```python
from build123d import *

# Parameters (mm, degrees)
SKETCH_R      = 1.5
SKETCH_W      = 56
SKETCH_H      = 40
PAD_DEPTH     = 3
SKETCH001_R   = 3
SKETCH001_R_2 = 1.5
PAD001_DEPTH  = 6
SKETCH002_R   = 2.25
POCKET_DEPTH  = 1.5


with BuildPart() as part:
    # Sketch → Pad (new body)
    with BuildSketch(Plane.XY):
        with BuildLine():
            Line((58, -3), (-4, -3))
            ThreePointArc((-7, 0), (-6.12132, -2.12132), (-4, -3))
            Line((-7, 0), (-7, 79))
            ThreePointArc((-1, 79), (-4, 82), (-7, 79))
            Line((-1, 79), (-1, 52))
            Line((-1, 52), (45, 52))
            Line((45, 52), (45, 79))
            ThreePointArc((51, 79), (48, 82), (45, 79))
            Line((51, 79), (51, 52))
            Line((51, 52), (58, 52))
            ThreePointArc((61, 49), (60.12132, 51.12132), (58, 52))
            Line((61, 0), (61, 49))
            ThreePointArc((58, -3), (60.12132, -2.12132), (61, 0))
        make_face()
        Circle(SKETCH_R, mode=Mode.SUBTRACT)
        with Locations((58, 0)):
            Circle(SKETCH_R, mode=Mode.SUBTRACT)
        with Locations((0, 49)):
            Circle(SKETCH_R, mode=Mode.SUBTRACT)
        with Locations((58, 49)):
            Circle(SKETCH_R, mode=Mode.SUBTRACT)
        with Locations((-4, 3)):
            Circle(SKETCH_R, mode=Mode.SUBTRACT)
        with Locations((48, 3)):
            Circle(SKETCH_R, mode=Mode.SUBTRACT)
        with Locations((48, 79)):
            Circle(SKETCH_R, mode=Mode.SUBTRACT)
        with Locations((-4, 79)):
            Circle(SKETCH_R, mode=Mode.SUBTRACT)
        with Locations((27, 26)):
            Rectangle(SKETCH_W, SKETCH_H, mode=Mode.SUBTRACT)
    extrude(amount=PAD_DEPTH)

    # Sketch001 (on Face27 of Pad) → Pad001 (join)
    with BuildSketch(Plane.XY.offset(3)):
        with Locations((-4, 79)):
            Circle(SKETCH001_R)
        with Locations((-4, 79)):
            Circle(SKETCH001_R_2, mode=Mode.SUBTRACT)
        with Locations((48, 79)):
            Circle(SKETCH001_R)
        with Locations((48, 79)):
            Circle(SKETCH001_R_2, mode=Mode.SUBTRACT)
        with Locations((48, 3)):
            Circle(SKETCH001_R)
        with Locations((48, 3)):
            Circle(SKETCH001_R_2, mode=Mode.SUBTRACT)
        with Locations((-4, 3)):
            Circle(SKETCH001_R)
        with Locations((-4, 3)):
            Circle(SKETCH001_R_2, mode=Mode.SUBTRACT)
    extrude(amount=PAD001_DEPTH)

    # Sketch002 (on Face5 of Pad001) → Pocket (cut)
    with BuildSketch(Plane.XY.offset(3)):
        Circle(SKETCH002_R)
        with Locations((58, 0)):
            Circle(SKETCH002_R)
        with Locations((58, 49)):
            Circle(SKETCH002_R)
        with Locations((0, 49)):
            Circle(SKETCH002_R)
    extrude(amount=-POCKET_DEPTH, mode=Mode.SUBTRACT)


solid = part.part
```
For this review, take the finished solid that the model builds, in its own axes (mm). A direction names the side the tool comes from. Give positions to 0.01 mm unless a question says otherwise; leave off trailing zeros. Order: outer loops, then holes, each group sorted by start corner. A loop starts at its lowest first (then second) coordinate and runs counter-clockwise, first axis right, second up.
1) Insertion check: pin 1 (3.5 mm diameter, centred on x = 18.5, z = 1.5, fed in from +Y); pin 2 (0.9 mm diameter, centred on y = 62.5, z = 1.5, fed in from +X); pin 3 (3.5 mm diameter, centred on x = 0.5, y = 49.5, fed in from +Z). Each pin has a flat end and moves straight along its axis. Give the tip position at first contact, or say it passes through.
2) The part is to be moulded in two halves that separate along Y. For faces 6 (the face through (46.89, 80.01, 4.44)), 7 (the face through (49.3, 1.7, 9)), 8 (the face through (-3.31, 1.67, 4.44)), 9 (the face through (-6.14, -2.1, 1.48)), say which applies: released by +Y, released by -Y, zero draft, split by the parting line, or undercut.
3) Take a section at C-C (x = 0). Give the boundary of the cut face in (y, z), then the cut area to 3 significant figures.
4) Take a section at B-B (y = 38). Give the boundary of the cut face in (x, z), then the cut area to 3 significant figures.
5) Take a section at D-D (x = 19.5). Give the boundary of the cut face in (y, z).
6) Take a section at A-A (z = 5.25). Give the boundary of the cut face in (x, y).
7) For faces 1 (the face through (27, 46, 1)), 2 (the face through (54, 52, 1)), 3 (the face through (0, 51, 1.5)), 4 (the face through (49.3, 77.7, 9)), 5 (the face through (-1, 66, 1)), list the 3-axis set-ups (+Z, -Z, +X, -X, +Y, -Y) from which the entire face can be reached by the end or side of a thin tool; tool diameter is ignored.
8) Wall thickness on line 1 (X direction, y = 79, z = 3.5); line 2 (Y direction, x = 0, z = 0.75); line 3 (X direction, y = 54.5, z = 1.5): over which ranges is each line inside the solid? List them lowest first.
Derived:
1. pin 1: stops at y = 52
1. pin 2: stops at x = 51
1. pin 3: stops at z = 3
2. face 6: undercut
2. face 7: zero draft
2. face 8: undercut
2. face 9: released by -Y
3. outline: (-3, 0) - (-1.5, 0) - (-1.5, 1.5) - (-2.25, 1.5) - (-2.25, 3) - (-3, 3) - close; (1.5, 0) - (6, 0) - (6, 3) - (2.25, 3) - (2.25, 1.5) - (1.5, 1.5) - close; (46, 0) - (47.5, 0) - (47.5, 1.5) - (46.75, 1.5) - (46.75, 3) - (46, 3) - close; (50.5, 0) - (52, 0) - (52, 3) - (51.25, 3) - (51.25, 1.5) - (50.5, 1.5) - close
3. area: 22.5 mm2
4. outline: (-7, 0) - (-1, 0) - (-1, 3) - (-7, 3) - close; (55, 0) - (61, 0) - (61, 3) - (55, 3) - close
4. area: 36.0 mm2
5. outline: (-3, 0) - (6, 0) - (6, 3) - (-3, 3) - close; (46, 0) - (52, 0) - (52, 3) - (46, 3) - close
6. outline: circle Ø6 at (-4, 3); circle Ø6 at (-4, 79); circle Ø6 at (48, 3); circle Ø6 at (48, 79); hole circle Ø3 at (-4, 3); hole circle Ø3 at (-4, 79); hole circle Ø3 at (48, 3); hole circle Ø3 at (48, 79)
7. face 1: +Z, -Z
7. face 2: +Z, -Z, +X, +Y
7. face 3: +Z
7. face 4: +Z, +X, -X, +Y, -Y
7. face 5: +Z, -Z, +Y
8. line 1: x = -7 to -5.5, -2.5 to -1, 45 to 46.5, 49.5 to 51
8. line 2: y = -3 to -1.5, 1.5 to 6, 46 to 47.5, 50.5 to 52
8. line 3: x = -7 to -1, 45 to 51
